Build history of the part. All positions in model axes, mm. Face numbers are marked on the shaded views. A direction names the side the tool comes from. Coordinates: 2 decimals unless noted, no trailing zeros. Order: outer loops, then holes, each group sorted by start corner. A loop starts at its lowest first (then second) coordinate and runs counter-clockwise, first axis right, second up. Notation, with made-up numbers: (-9, -18) - (50, -18) arc R26 ccw to (50, 19) - close; hole circle Ø11 at (-13.5, 83). An arc over 180 degrees is marked (long way). Return JSON: item names as keys, results as strings.
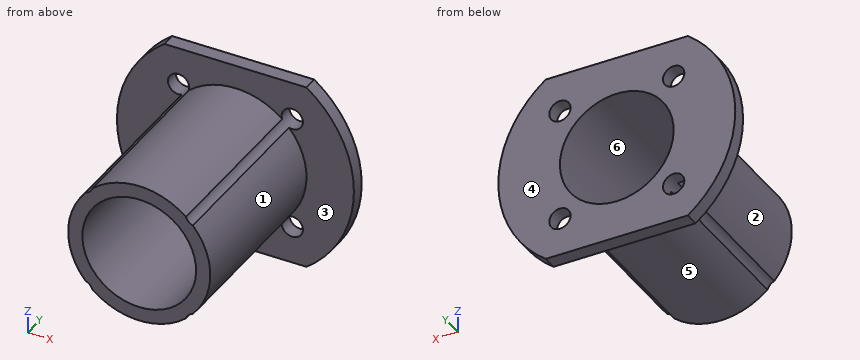
from build123d import *

# Parameters (mm, degrees)
CUT_EXTRUDE3_START   = 37
CUT_EXTRUDE3_DEPTH   = 3
M4_CLEARANCE_HOLE1_D = 4.5


# Read off the part's stored shape, not the designer's step: Cut-Extrude3
with BuildPart() as part:
    # Sketch1 → Revolve1 (revolve)
    with BuildSketch(Plane.XY, mode=Mode.PRIVATE) as revolve1_sk:
        Polygon((12, 40), (12, 0), (15, 0), (15, 37), (25, 37), (25, 40), align=None)
    revolve(revolve1_sk.sketch.rotate(Axis((0, 0, 0), (0, 1, 0)), 90), axis=Axis((0, 0, 0), (0, 1, 0)))

    # Cut-Extrude3 outline → Cut-Extrude3 (cut)
    with BuildSketch(Plane(origin=(0, 0, 0), x_dir=(1, 0, 0), z_dir=(0, 1, 0)).offset(CUT_EXTRUDE3_START)):
        with BuildLine():
            Line((15, -20), (-15, -20))
            ThreePointArc((-15, -20), (0, -25), (15, -20))
        make_face()
        with BuildLine():
            ThreePointArc((15, 20), (0, 25), (-15, 20))
            Line((-15, 20), (15, 20))
        make_face()
    extrude(amount=CUT_EXTRUDE3_DEPTH, mode=Mode.SUBTRACT)

    # M4 Clearance Hole1 (through all)
    with Locations(Plane(origin=(0, 40, 0), x_dir=(1, 0, 0), z_dir=(0, 1, 0))):
        with Locations((-12, 12), (12, 12), (12, -12), (-12, -12), (0, 0)):
            Hole(M4_CLEARANCE_HOLE1_D / 2)


solid = part.part
1. Cut at C-C on y = 25. Give the cut face in (x, z), plus the area to 3 significant figures.
Check values:
{"outline": "(-11.3, -9.86) arc R2.25 cw to (-9.86, -11.3) arc R15 ccw to (9.86, -11.3) arc R2.25 cw to (11.3, -9.86) arc R15 ccw to (11.3, 9.86) arc R2.25 cw to (9.86, 11.3) arc R15 ccw to (-9.86, 11.3) arc R2.25 cw to (-11.3, 9.86) arc R15 ccw to start; hole circle Ø24 at (0, 0)", "area": "253 mm²"}
2. Cut at B-B on z = 0. Give the cut face in (x, y).
Check values:
{"outline": "(-25, 37) - (-15, 37) - (-15, 0) - (-12, 0) - (-12, 40) - (-25, 40) - close; (12, 0) - (15, 0) - (15, 37) - (25, 37) - (25, 40) - (12, 40) - close"}
3. Cut at A-A on x = 0. Give the cut face in (y, z), plus the area to 3 significant figures.
Check values:
{"outline": "(0, -15) - (37, -15) - (37, -20) - (40, -20) - (40, -12) - (0, -12) - close; (0, 12) - (40, 12) - (40, 20) - (37, 20) - (37, 15) - (0, 15) - close", "area": "270 mm²"}
4. Tool access for the marked faces 1, 2 and 3: list every direction of +Z, -Z, +X, -X, +Y, -Y with a clear straight run to the whole face (end or side of a thin tool).
Check values:
{"face 1": "+X, -Y", "face 2": "-X, -Y", "face 3": "-Y"}
5. Cut at D-D on z = -17. Give the cut face in (x, y).
Check values:
{"outline": "(-18.33, 37) - (18.33, 37) - (18.33, 40) - (-18.33, 40) - close"}
6. Drop flat-ended pins along their axis: pin 1 (10 mm diameter, centred on x = 18.5, y = 18, fed in from -Z); pin 2 (3.5 mm diameter, centred on x = 12, z = -12, fed in from +Y); pin 3 (6 mm diameter, centred on x = 13, y = 25.5, fed in from +Z); pin 4 (3 mm diameter, centred on y = 21.5, z = 2, fed in from +X). Give the stop position or say it passes through.
Check values:
{"pin 1": "z = -6.54", "pin 2": "through", "pin 3": "z = 10.97", "pin 4": "x = 14.99"}
7. Probe L1, parallel to X at y = 31, z = 0.5; L2, parallel to Y at x = 20, z = -8.5; L3, parallel to X at y = 23.5, z = -1.5. List the from-to ranges inside material, lowest first.
Check values:
{"L1": "-14.99 to -11.99, 11.99 to 14.99", "L2": "37 to 40", "L3": "-14.92 to -11.91, 11.91 to 14.92"}
8. Mould opens along Z. For the marked faces 4, 5 and 6 say: pulls with the +Z half, pulls with the -Z half, needs draft (parallel to the pull), parting line crosses it, or undercut.
Check values:
{"face 4": "needs draft", "face 5": "pulls with the -Z half", "face 6": "undercut"}
